from build123d import *

# Parameters (mm, degrees)
F0_W     = 40
F0_H     = 5
F0_W_2   = 20.0747972727
F0_W_3   = 19.9252027273
F1_DEPTH = 2
F2_R     = 0.99999
F3_R     = 0.99999
F4_R     = 0.99999


# Not quite as in the source:
# - a fillet or chamfer is up to 0.001 mm smaller than in the source, because OpenCascade refuses the exact size


with BuildPart() as f1:
    # F0 (on Front) → F1 (new body)
    with BuildSketch(Plane.XZ):
        Polygon((-17.9821681231, 15), (-20, 15), (-20, 2.6505640079), (20, 2.6505640079), (20, 15), (18.0178318769, 15), (18.0178318769, 13), (-17.9821681231, 13), align=None)
        with Locations((0, 0.1505640079)):
            Rectangle(F0_W, F0_H)
        with Locations((30.0373986363, 0.1505640079)):
            Rectangle(F0_W_2, F0_H)
        with Locations((-29.9626013637, 0.1505640079)):
            Rectangle(F0_W_3, F0_H)
        Polygon((20, -2.3494359921), (-20, -2.3494359921), (-20, -15), (-18.0797521025, -15), (-18.0797521025, -13), (17.9202478975, -13), (17.9202478975, -15), (20, -15), align=None)
    extrude(amount=F1_DEPTH)

    # F2 (radius 1 in the source; OpenCascade refuses exactly that, so slightly less here)
    f2_edges = [f1.edges().sort_by_distance(p)[0] for p in [
        (30.037399, -2, -2.349436),
        (30.037399, 0, -2.349436),
        (30.037399, -2, 2.650564),
        (-29.962601, 0, 2.650564),
        (-29.962601, -2, 2.650564),
        (-29.962601, 0, -2.349436),
        (30.037399, 0, 2.650564),
        (-29.962601, -2, -2.349436),
    ]]
    fillet(f2_edges, radius=F2_R)

    # F3 (radius 1 in the source; OpenCascade refuses exactly that, so slightly less here)
    f3_edges = [f1.edges().sort_by_distance(p)[0] for p in [
        (-0.079752, -2, -13),
        (-0.079752, 0, -13),
        (0.017832, 0, 13),
        (0.017832, -2, 13),
    ]]
    fillet(f3_edges, radius=F3_R)

    # F4 (radius 1 in the source; OpenCascade refuses exactly that, so slightly less here)
    f4_edges = [f1.edges().sort_by_distance(p)[0] for p in [
        (18.017832, -2, 14),
        (18.017832, -1, 15),
        (18.017832, 0, 14),
        (-17.982168, -2, 14),
        (-17.982168, -1, 15),
        (-18.079752, -2, -14),
        (17.920248, -2, -14),
        (-17.982168, 0, 14),
        (-18.079752, 0, -14),
        (-18.079752, -1, -15),
        (17.920248, 0, -14),
        (17.920248, -1, -15),
    ]]
    fillet(f4_edges, radius=F4_R)


solid = f1.part
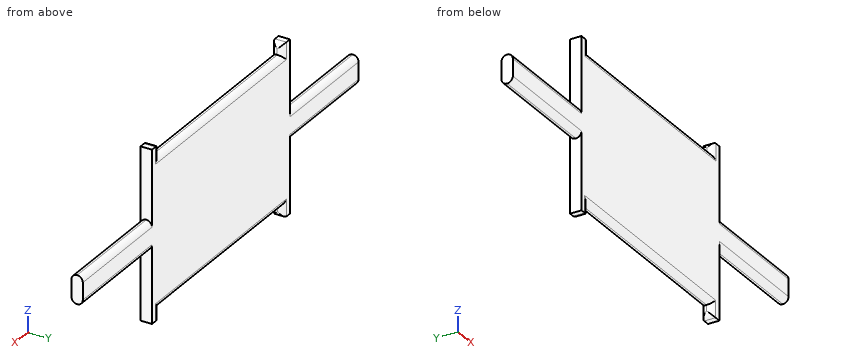
Design review of the part built by this model. Coordinates are the model's own, in mm. Coordinates: 2 decimals unless noted, no trailing zeros. Loops run counter-clockwise (first coordinate to the right, second up) from the corner with the lowest first, then second, coordinate; pieces in that order, holes last. Notation, with made-up numbers: (-14, 29) -> (-7, 29) arc R25 ccw to (-7, 51) -> close; hole circle Ø10 at (64, -28.75). An arc over 180 degrees is marked (long way). Use a Markdown table: item, result. Add a question column.
Item 1: Clearance check with flat-ended pins moving along their axes: P1, Ø1, axis at x = -22.5, y = -1, coming from the +Z side; P2, Ø1, axis at y = -1, z = 10, coming from the -X side. State where each tip first meets the part, or that it passes through.
Item 2: Wall thickness on L1, parallel to X at y = -0.9, z = 11; L2, parallel to X at y = -0.3, z = 12.75; L3, parallel to Z at x = 30.5, y = -1: over which ranges is each line inside the solid? List them lowest first. Write a range as from..to.
Item 3: We need section C-C, the plane z = -8.5. Write out the cut boundary in (x, y), and give its area (3 significant figures).
Item 4: We need section B-B, the plane y = -0.55. Write out the cut boundary in (x, z).
Numbers:
| question | item | result |
|---|---|---|
| 1 | P1 | stops at z = 2.65 |
| 1 | P2 | stops at x = -20 |
| 2 | L1 | x = -20..20 |
| 2 | L2 | x = -20..-18.27, 18.3..20 |
| 2 | L3 | z = -2.35..2.65 |
| 3 | outline | (-20, -2) -> (20, -2) -> (20, 0) -> (-20, 0) -> close |
| 3 | area | 80.0 mm^2 |
| 4 | outline | (-39.93, -2.24) -> (-20, -2.24) -> (-20, -15) -> (-19.08, -15) arc R1 ccw to (-18.19, -14.45) -> (-18.19, -12.89) -> (18.03, -12.89) -> (18.03, -14.45) arc R1 ccw to (18.92, -15) -> (20, -15) -> (20, -2.24) -> (40.07, -2.24) -> (40.07, 2.54) -> (20, 2.54) -> (20, 15) -> (19.02, 15) arc R1 ccw to (18.12, 14.45) -> (18.12, 12.89) -> (-18.09, 12.89) -> (-18.09, 14.45) arc R1 ccw to (-18.98, 15) -> (-20, 15) -> (-20, 2.54) -> (-39.93, 2.54) -> close |
